Could you check a few things on this model? Use its own coordinates, in mm. A direction names the side the tool comes from. Give positions to 0.01 mm unless a question says otherwise; leave off trailing zeros. Write each loop counter-clockwise with the first axis right and the second up, starting at its lowest first coordinate (ties: lowest second). Pieces come first, ordered by that corner, then holes. Notation, with made-up numbers: (35.25, 14.25) - (74.25, 14.25) arc R16 ccw to (74.25, 19.25) - close; hole circle Ø6 at (-6, 28). An arc over 180 degrees is marked (long way). Write item = value, one per line.
from build123d import *

# Parameters (mm, degrees)
SKETCH1_R               = 2.6035
BOSS_EXTRUDE1_DEPTH     = 457.2
CUT_EXTRUDE2_DEPTH      = 4.318
CUT_EXTRUDE2_DEPTH_BACK = 26.924


with BuildPart() as part:
    # Sketch1 → Boss-Extrude1 (new body, symmetric)
    with BuildSketch(Plane.XY):
        with BuildLine():
            Line((-7.179650497, -8.645192506), (-3.952270251, -5.423690499))
            ThreePointArc((-3.952270251, -5.423690499), (-2.922936451, -4.736929036), (-1.709253557, -4.4958))
            Line((-1.709253557, -4.4958), (1.709253557, -4.4958))
            ThreePointArc((1.709253557, -4.4958), (2.922936451, -4.736929036), (3.952270251, -5.423690499))
            Line((3.952270251, -5.423690499), (7.179650497, -8.645192506))
            ThreePointArc((7.179650497, -8.645192506), (7.41473083, -9.822813117), (6.416408329, -10.4902))
            Line((6.416408329, -10.4902), (4.287512407, -10.4902))
            ThreePointArc((4.287512407, -10.4902), (3.54574862, -10.79744862), (3.2385, -11.539212407))
            Line((3.2385, -11.539212407), (3.2385, -11.650987593))
            ThreePointArc((3.2385, -11.650987593), (3.54574862, -12.39275138), (4.287512407, -12.7))
            Line((4.287512407, -12.7), (5.317126718, -12.7))
            ThreePointArc((5.317126718, -12.7), (5.825126718, -12.192), (6.333126718, -12.7))
            Line((6.333126718, -12.7), (9.550443118, -12.7))
            ThreePointArc((9.550443118, -12.7), (10.058366869, -12.192000006), (10.566443095, -12.699847501))
            ThreePointArc((10.566443095, -12.699847501), (12.082537762, -12.08250727), (12.699846982, -10.566399977))
            ThreePointArc((12.699846982, -10.566399977), (12.192000006, -10.058323491), (12.7, -9.5504))
            Line((12.7, -9.5504), (12.7, -6.3330836))
            ThreePointArc((12.7, -6.3330836), (12.192, -5.8250836), (12.7, -5.3170836))
            Line((12.7, -5.3170836), (12.7, -4.287469289))
            ThreePointArc((12.7, -4.287469289), (12.39275138, -3.545705502), (11.650987593, -3.238456882))
            Line((11.650987593, -3.238456882), (11.539212407, -3.238456882))
            ThreePointArc((11.539212407, -3.238456882), (10.79744862, -3.545705502), (10.4902, -4.287469289))
            Line((10.4902, -4.287469289), (10.4902, -6.402089023))
            ThreePointArc((10.4902, -6.402089023), (9.856505071, -7.351067942), (8.737131347, -7.129408934))
            Line((8.737131347, -7.129408934), (5.441005833, -3.840816462))
            ThreePointArc((5.441005833, -3.840816462), (4.750877967, -2.809883091), (4.5085, -1.593185507))
            Line((4.5085, -1.593185507), (4.5085, 1.593185507))
            ThreePointArc((4.5085, 1.593185507), (4.750877967, 2.809883091), (5.441005833, 3.840816462))
            Line((5.441005833, 3.840816462), (8.737131347, 7.129408934))
            ThreePointArc((8.737131347, 7.129408934), (9.856505071, 7.351067942), (10.4902, 6.402089023))
            Line((10.4902, 6.402089023), (10.4902, 4.287469289))
            ThreePointArc((10.4902, 4.287469289), (10.79744862, 3.545705502), (11.539212407, 3.238456882))
            Line((11.539212407, 3.238456882), (11.650987593, 3.238456882))
            ThreePointArc((11.650987593, 3.238456882), (12.39275138, 3.545705502), (12.7, 4.287469289))
            Line((12.7, 4.287469289), (12.7, 5.3170836))
            ThreePointArc((12.7, 5.3170836), (12.192, 5.8250836), (12.7, 6.3330836))
            Line((12.7, 6.3330836), (12.7, 9.5504))
            ThreePointArc((12.7, 9.5504), (12.192000006, 10.058323491), (12.699846982, 10.566399977))
            ThreePointArc((12.699846982, 10.566399977), (12.082537762, 12.08250727), (10.566443095, 12.699847501))
            ThreePointArc((10.566443095, 12.699847501), (10.058366869, 12.192000006), (9.550443118, 12.7))
            Line((9.550443118, 12.7), (6.333126718, 12.7))
            ThreePointArc((6.333126718, 12.7), (5.825126718, 12.192), (5.317126718, 12.7))
            Line((5.317126718, 12.7), (4.287512407, 12.7))
            ThreePointArc((4.287512407, 12.7), (3.54574862, 12.39275138), (3.2385, 11.650987593))
            Line((3.2385, 11.650987593), (3.2385, 11.539212407))
            ThreePointArc((3.2385, 11.539212407), (3.54574862, 10.79744862), (4.287512407, 10.4902))
            Line((4.287512407, 10.4902), (6.476788598, 10.4902))
            ThreePointArc((6.476788598, 10.4902), (7.432222385, 9.85140422), (7.207036008, 8.724370562))
            Line((7.207036008, 8.724370562), (3.898272566, 5.423169045))
            ThreePointArc((3.898272566, 5.423169045), (2.869120213, 4.736787962), (1.655778399, 4.4958))
            Line((1.655778399, 4.4958), (-1.655778399, 4.4958))
            ThreePointArc((-1.655778399, 4.4958), (-2.869120213, 4.736787962), (-3.898272566, 5.423169045))
            Line((-3.898272566, 5.423169045), (-7.207036008, 8.724370562))
            ThreePointArc((-7.207036008, 8.724370562), (-7.432222385, 9.85140422), (-6.476788598, 10.4902))
            Line((-6.476788598, 10.4902), (-4.287512407, 10.4902))
            ThreePointArc((-4.287512407, 10.4902), (-3.54574862, 10.79744862), (-3.2385, 11.539212407))
            Line((-3.2385, 11.539212407), (-3.2385, 11.650987593))
            ThreePointArc((-3.2385, 11.650987593), (-3.54574862, 12.39275138), (-4.287512407, 12.7))
            Line((-4.287512407, 12.7), (-5.317126718, 12.7))
            ThreePointArc((-5.317126718, 12.7), (-5.825126718, 12.192), (-6.333126718, 12.7))
            Line((-6.333126718, 12.7), (-9.550443118, 12.7))
            ThreePointArc((-9.550443118, 12.7), (-10.058366869, 12.192000006), (-10.566443095, 12.699847501))
            ThreePointArc((-10.566443095, 12.699847501), (-12.082537762, 12.08250727), (-12.699846982, 10.566399977))
            ThreePointArc((-12.699846982, 10.566399977), (-12.192000006, 10.058323491), (-12.7, 9.5504))
            Line((-12.7, 9.5504), (-12.7, 6.3330836))
            ThreePointArc((-12.7, 6.3330836), (-12.192, 5.8250836), (-12.7, 5.3170836))
            Line((-12.7, 5.3170836), (-12.7, 4.287469289))
            ThreePointArc((-12.7, 4.287469289), (-12.39275138, 3.545705502), (-11.650987593, 3.238456882))
            Line((-11.650987593, 3.238456882), (-11.539212407, 3.238456882))
            ThreePointArc((-11.539212407, 3.238456882), (-10.79744862, 3.545705502), (-10.4902, 4.287469289))
            Line((-10.4902, 4.287469289), (-10.4902, 6.402089023))
            ThreePointArc((-10.4902, 6.402089023), (-9.856505071, 7.351067942), (-8.737131347, 7.129408934))
            Line((-8.737131347, 7.129408934), (-5.441005833, 3.840816462))
            ThreePointArc((-5.441005833, 3.840816462), (-4.750877967, 2.809883091), (-4.5085, 1.593185507))
            Line((-4.5085, 1.593185507), (-4.5085, -1.593185507))
            ThreePointArc((-4.5085, -1.593185507), (-4.750877967, -2.809883091), (-5.441005833, -3.840816462))
            Line((-5.441005833, -3.840816462), (-8.737131347, -7.129408934))
            ThreePointArc((-8.737131347, -7.129408934), (-9.856505071, -7.351067942), (-10.4902, -6.402089023))
            Line((-10.4902, -6.402089023), (-10.4902, -4.287469289))
            ThreePointArc((-10.4902, -4.287469289), (-10.79744862, -3.545705502), (-11.539212407, -3.238456882))
            Line((-11.539212407, -3.238456882), (-11.650987593, -3.238456882))
            ThreePointArc((-11.650987593, -3.238456882), (-12.39275138, -3.545705502), (-12.7, -4.287469289))
            Line((-12.7, -4.287469289), (-12.7, -5.3170836))
            ThreePointArc((-12.7, -5.3170836), (-12.192, -5.8250836), (-12.7, -6.3330836))
            Line((-12.7, -6.3330836), (-12.7, -9.5504))
            ThreePointArc((-12.7, -9.5504), (-12.192000006, -10.058323491), (-12.699846982, -10.566399977))
            ThreePointArc((-12.699846982, -10.566399977), (-12.082537762, -12.08250727), (-10.566443095, -12.699847501))
            ThreePointArc((-10.566443095, -12.699847501), (-10.058366869, -12.192000006), (-9.550443118, -12.7))
            Line((-9.550443118, -12.7), (-6.333126718, -12.7))
            ThreePointArc((-6.333126718, -12.7), (-5.825126718, -12.192), (-5.317126718, -12.7))
            Line((-5.317126718, -12.7), (-4.287512407, -12.7))
            ThreePointArc((-4.287512407, -12.7), (-3.54574862, -12.39275138), (-3.2385, -11.650987593))
            Line((-3.2385, -11.650987593), (-3.2385, -11.539212407))
            ThreePointArc((-3.2385, -11.539212407), (-3.54574862, -10.79744862), (-4.287512407, -10.4902))
            Line((-4.287512407, -10.4902), (-6.416408329, -10.4902))
            ThreePointArc((-6.416408329, -10.4902), (-7.41473083, -9.822813117), (-7.179650497, -8.645192506))
        make_face()
        Circle(SKETCH1_R, mode=Mode.SUBTRACT)
    extrude(amount=BOSS_EXTRUDE1_DEPTH, both=True)

    # Sketch3 → Cut-Extrude2 (cut, two sides)
    with BuildSketch(Plane.ZY.offset(12.7)) as cut_extrude2_sk:
        Polygon((-203.2, 21.063041056), (-461.090893327, 21.063041056), (-461.090893327, -25.4), (-203.2, -27.249602883), (257.029766368, -27.249602883), (257.029766368, 21.063041056), align=None)
    extrude(amount=CUT_EXTRUDE2_DEPTH, mode=Mode.SUBTRACT)
    extrude(cut_extrude2_sk.sketch, amount=-CUT_EXTRUDE2_DEPTH_BACK, mode=Mode.SUBTRACT)


solid = part.part
1. Thinking about a two-plate mould opening in Y: for faces 1 (the face through (4.508, 0, 359)), 2 (the face through (-7.112, 5.508, 358.516)), 3 (the face through (-8, -12.7, 359)), 4 (the face through (8, 12.7, 359)), which applies, pulls with the +Y half, pulls with the -Y half, needs draft (parallel to the pull), parting line crosses it, or undercut?
Filled sheet:
face_1 = undercut
face_2 = undercut
face_3 = pulls with the -Y half
face_4 = pulls with the +Y half
2. If we section it at A-A, the plane x = 0: Please give me the cut outline in (y, z), and give its area (3 significant figures).
Filled sheet:
outline = (-4.5, 257.03) - (-2.6, 257.03) - (-2.6, 457.2) - (-4.5, 457.2) - close; (2.6, 257.03) - (4.5, 257.03) - (4.5, 457.2) - (2.6, 457.2) - close
area = 758 mm2
3. I need wall thicknesses on line 1 (X direction, y = 9.25, z = 373); line 2 (Y direction, x = -6.75, z = 404); line 3 (X direction, y = 0, z = 309). Which ranges of each line are inside material? Lowest first, please.
Filled sheet:
line_1 = -12.7 to -7.49, 7.49 to 12.7
line_2 = -12.7 to -10.44, -8.22 to -5.15, 5.15 to 8.27, 10.45 to 12.7
line_3 = -4.51 to -2.6, 2.6 to 4.51
4. For pin 1 (3 mm diameter, centred on y = 1, z = 429, fed in from -X); pin 2 (4 mm diameter, centred on x = 1.5, z = 385.5, fed in from -Y); pin 3 (1.6 mm diameter, centred on y = 0.5, z = 322, fed in from -X), each with a flat end and sliding along its axis, tell me the tip position at first contact or that it passes through.
Filled sheet:
pin_1 = -4.64
pin_2 = -12.34
pin_3 = -4.51
5. Which directions (+Z, -Z, +X, -X, +Y, -Y) give clear straight access to the entire face, cutting with the end or side of a thin tool? Please do faces 5 (the face through (0, 4.496, 359)), 6 (the face through (-12.7, -8, 359)), 7 (the face through (0, -4.496, 359)), 8 (the face through (-5.59, -7.06, 358.52)).
Filled sheet:
face_5 = +Z, -Z, +Y
face_6 = +Z, -Z, -X, +Y, -Y
face_7 = +Z, -Z, -Y
face_8 = +Z, -Z
